from build123d import *

# Parameters (mm, degrees)
SKETCH_1_R          = 2
EXTRUDE_1_DEPTH     = 5
SKETCH_2_W          = 60
SKETCH_2_H          = 24.578099901
SKETCH_2_W_2        = 20
SKETCH_2_H_2        = 18.209440524
CUT_EXTRUDE_1_DEPTH = 29
FILLET_1_R          = 3


with BuildPart() as part:
    # 草图1 → 凸台-拉伸1 (new body)
    with BuildSketch(Plane.XY):
        with BuildLine():
            Line((-85, 0), (85, 0))
            Line((85, 0), (85, -38))
            ThreePointArc((85, -38), (82.071067812, -45.071067812), (75, -48))
            Line((75, -48), (-75, -48))
            ThreePointArc((-75, -48), (-82.071067812, -45.071067812), (-85, -38))
            Line((-85, -38), (-85, 0))
        make_face()
        with Locations((-80, -11)):
            Circle(SKETCH_1_R, mode=Mode.SUBTRACT)
        with Locations((0, -11)):
            Circle(SKETCH_1_R, mode=Mode.SUBTRACT)
        with Locations((80, -11)):
            Circle(SKETCH_1_R, mode=Mode.SUBTRACT)
        with Locations((-80, -36.5)):
            Circle(SKETCH_1_R, mode=Mode.SUBTRACT)
        with Locations((80, -36.5)):
            Circle(SKETCH_1_R, mode=Mode.SUBTRACT)
        with Locations((-26.666666667, -36.5)):
            Circle(SKETCH_1_R, mode=Mode.SUBTRACT)
        with Locations((26.666666667, -36.5)):
            Circle(SKETCH_1_R, mode=Mode.SUBTRACT)
    extrude(amount=EXTRUDE_1_DEPTH)

    # 草图2 → 切除-拉伸1 (cut)
    with BuildSketch(Plane.XY):
        with Locations((-45, -0.145574748)):
            Rectangle(SKETCH_2_W, SKETCH_2_H)
        with Locations((65, -5.064712671)):
            Rectangle(SKETCH_2_W_2, SKETCH_2_H_2)
    extrude(amount=CUT_EXTRUDE_1_DEPTH, mode=Mode.SUBTRACT)

    # 圆角1
    fillet_1_edges = [part.edges().sort_by_distance(p)[0] for p in [
        (-85, 0, 2.5),
        (85, 0, 2.5),
        (55, 0, 2.5),
        (75, 0, 2.5),
        (-75, 0, 2.5),
        (-15, 0, 2.5),
        (-75, -12.434624699, 2.5),
        (-15, -12.434624699, 2.5),
        (55, -14.169432933, 2.5),
        (75, -14.169432933, 2.5),
    ]]
    fillet(fillet_1_edges, radius=FILLET_1_R)


solid = part.part
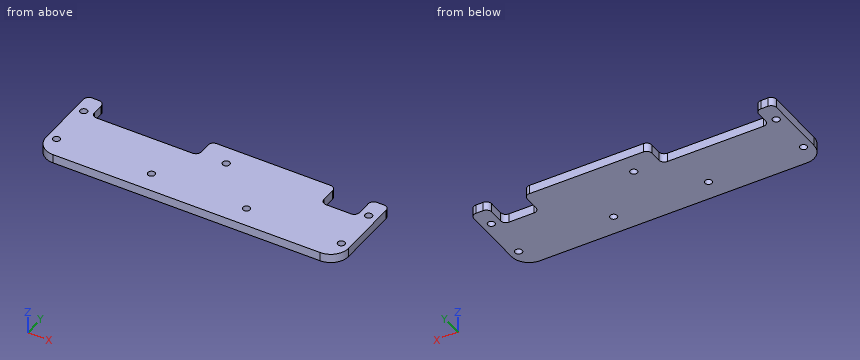
The model under review builds one solid part; all positions refer to its coordinate system, in mm. Coordinates: 2 decimals unless noted, no trailing zeros. Write each loop counter-clockwise with the first axis right and the second up, starting at its lowest first coordinate (ties: lowest second). Pieces come first, ordered by that corner, then holes. Notation, with made-up numbers: (87, 65.25) -> (92, 65.25) arc R27 cw to (92, 97.25) -> close; hole circle Ø10 at (9, 82). An arc over 180 degrees is marked (long way). Answer in a Markdown table with one row per item.
1. We need section B-B, the plane z = 1.1. Give the number of separate pieces and of enclosed holes in the cut face, and give its area (3 significant figures).
Answers below:
| item | result |
|---|---|
| separate pieces | 1 |
| enclosed holes | 7 |
| area | 7,000 mm^2 |
2. Wall thickness on probe 1 along X at (y, z) = (-7, 3.05); probe 2 along X at (y, z) = (-12.5, 3.3); probe 3 along Y at (x, z) = (0, 2.15): over which ranges is each line inside the solid? List them lowest first. Write a range as [from, to].
Answers below:
| item | result |
|---|---|
| probe 1 | x = [-85, -75], [-15, 55], [75, 85] |
| probe 2 | x = [-85, -81.32], [-78.68, -1.32], [1.32, 55.31], [74.69, 78.68], [81.32, 85] |
| probe 3 | y = [-48, -13], [-9, 0] |
3. Clearance check with flat-ended pins moving along their axes: pin 1 Ø3 at (x, y) = (80, -11) entering from -Z (3 decimals); pin 2 Ø2 at (x, z) = (68, 2.5) entering from +Y; pin 3 Ø1 at (x, z) = (53.5, 2) entering from +Y; pin 4 Ø5 at (x, y) = (-80, -36.5) entering from -Z. State where each tip first meets the part, or that it passes through.
Answers below:
| item | result |
|---|---|
| pin 1 | passes through |
| pin 2 | stops at y = -14.17 |
| pin 3 | stops at y = -0.17 |
| pin 4 | stops at z = 0 |
4. We need section D-D, the plane x = 80. State the section outline as (y, z) points, and give its area (3 significant figures).
Answers below:
| item | result |
|---|---|
| outline | (-46.66, 0) -> (-38.5, 0) -> (-38.5, 5) -> (-46.66, 5) -> close; (-34.5, 0) -> (-13, 0) -> (-13, 5) -> (-34.5, 5) -> close; (-9, 0) -> (0, 0) -> (0, 5) -> (-9, 5) -> close |
| area | 193 mm^2 |
5. We need section C-C, the plane x = 0. State the section outline as (y, z) points.
Answers below:
| item | result |
|---|---|
| outline | (-48, 0) -> (-13, 0) -> (-13, 5) -> (-48, 5) -> close; (-9, 0) -> (0, 0) -> (0, 5) -> (-9, 5) -> close |
6. We need section A-A, the plane y = -36.5. State the section outline as (x, z) points, and give its area (3 significant figures).
Answers below:
| item | result |
|---|---|
| outline | (-85, 0) -> (-82, 0) -> (-82, 5) -> (-85, 5) -> close; (-78, 0) -> (-28.67, 0) -> (-28.67, 5) -> (-78, 5) -> close; (-24.67, 0) -> (24.67, 0) -> (24.67, 5) -> (-24.67, 5) -> close; (28.67, 0) -> (78, 0) -> (78, 5) -> (28.67, 5) -> close; (82, 0) -> (85, 0) -> (85, 5) -> (82, 5) -> close |
| area | 770 mm^2 |
